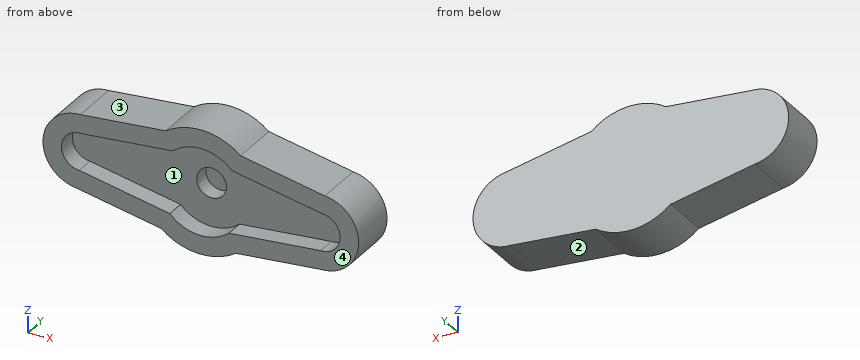
```python
from build123d import *

# Parameters (mm, degrees)
SKETCH1_R           = 2.032
BOSS_EXTRUDE1_DEPTH = 2.159
BOSS_EXTRUDE2_START = -2.54
BOSS_EXTRUDE2_DEPTH = 2.54
BOSS_EXTRUDE3_START = 2.159
BOSS_EXTRUDE3_DEPTH = 2


with BuildPart() as part:
    # Sketch1 → Boss-Extrude1 (new body)
    with BuildSketch(Plane(origin=(0, 19.05, 0), x_dir=(1, 0, 0), z_dir=(0, 1, 0))):
        with BuildLine():
            Line((27.891662372, 5.862371385), (16.22825993, 6.965475496))
            ThreePointArc((16.22825993, 6.965475496), (11.029140385, 8.448695687), (5.993806888, 6.479888246))
            Line((5.993806888, 6.479888246), (-5.512759891, 4.277454099))
            ThreePointArc((-5.512759891, 4.277454099), (-10.135739741, -1.023215233), (-5.031662372, -5.862371385))
            Line((-5.031662372, -5.862371385), (6.63174007, -6.965475496))
            ThreePointArc((6.63174007, -6.965475496), (11.830859615, -8.448695687), (16.866193112, -6.479888246))
            Line((16.866193112, -6.479888246), (28.372759891, -4.277454099))
            ThreePointArc((28.372759891, -4.277454099), (32.995739741, 1.023215233), (27.891662372, 5.862371385))
        make_face()
        with Locations(Location((11.43, 0, 0), (0, 0, 270))):
            Circle(SKETCH1_R, mode=Mode.SUBTRACT)
    extrude(amount=BOSS_EXTRUDE1_DEPTH)

    # Sketch1<3> → Boss-Extrude2 (add)
    with BuildSketch(Plane(origin=(0, 19.05, 0), x_dir=(1, 0, 0), z_dir=(0, 1, 0)).offset(BOSS_EXTRUDE2_START)):
        with BuildLine():
            Line((5.993806888, 6.479888246), (-5.512759891, 4.277454099))
            ThreePointArc((-5.512759891, 4.277454099), (-10.135739741, -1.023215233), (-5.031662372, -5.862371385))
            Line((-5.031662372, -5.862371385), (6.63174007, -6.965475496))
            ThreePointArc((6.63174007, -6.965475496), (11.830859615, -8.448695687), (16.866193112, -6.479888246))
            Line((16.866193112, -6.479888246), (28.372759891, -4.277454099))
            ThreePointArc((28.372759891, -4.277454099), (32.995739741, 1.023215233), (27.891662372, 5.862371385))
            Line((27.891662372, 5.862371385), (16.22825993, 6.965475496))
            ThreePointArc((16.22825993, 6.965475496), (11.029140385, 8.448695687), (5.993806888, 6.479888246))
        make_face()
        with BuildLine():
            ThreePointArc((28.0418263, -1.754687144), (30.458593889, 0.90283697), (27.801069775, 3.319604559))
            Line((27.801069775, 3.319604559), (15.268026397, 4.504957782))
            ThreePointArc((15.268026397, 4.504957782), (11.149518648, 5.911549835), (7.18268751, 4.121338114))
            Line((7.18268751, 4.121338114), (-5.1818263, 1.754687144))
            ThreePointArc((-5.1818263, 1.754687144), (-7.598593889, -0.90283697), (-4.941069775, -3.319604559))
            Line((-4.941069775, -3.319604559), (7.591973603, -4.504957782))
            ThreePointArc((7.591973603, -4.504957782), (11.710481352, -5.911549835), (15.67731249, -4.121338114))
            Line((15.67731249, -4.121338114), (28.0418263, -1.754687144))
        make_face(mode=Mode.SUBTRACT)
    extrude(amount=BOSS_EXTRUDE2_DEPTH)

    # Sketch1<4> → Boss-Extrude3 (add)
    with BuildSketch(Plane(origin=(0, 19.05, 0), x_dir=(1, 0, 0), z_dir=(0, 1, 0)).offset(BOSS_EXTRUDE3_START)):
        with BuildLine():
            Line((27.891662372, 5.862371385), (16.22825993, 6.965475496))
            ThreePointArc((16.22825993, 6.965475496), (11.029140385, 8.448695687), (5.993806888, 6.479888246))
            Line((5.993806888, 6.479888246), (-5.512759891, 4.277454099))
            ThreePointArc((-5.512759891, 4.277454099), (-10.135739741, -1.023215233), (-5.031662372, -5.862371385))
            Line((-5.031662372, -5.862371385), (6.63174007, -6.965475496))
            ThreePointArc((6.63174007, -6.965475496), (11.830859615, -8.448695687), (16.866193112, -6.479888246))
            Line((16.866193112, -6.479888246), (28.372759891, -4.277454099))
            ThreePointArc((28.372759891, -4.277454099), (32.995739741, 1.023215233), (27.891662372, 5.862371385))
        make_face()
    extrude(amount=BOSS_EXTRUDE3_DEPTH)


solid = part.part
```
Design review of the part built by this model. Coordinates are the model's own, in mm. Face numbers are marked on the shaded views. Give positions to 0.01 mm unless a question says otherwise; leave off trailing zeros. Order: outer loops, then holes, each group sorted by start corner. A loop starts at its lowest first (then second) coordinate and runs counter-clockwise, first axis right, second up. Notation, with made-up numbers: M -8.5,43 L 41.5,43 A9 ccw 41.5,59 Z; hole C 30.5,24 d3. An arc over 180 degrees is marked long. One line per question, with ' | ' between items. Start each with the question number.
Q1. We need section A-A (y = 19.5). Write out the cut boundary in (x, z).
Q2. For L1, parallel to Y at x = 27, z = 1.75; L2, parallel to Z at x = 5, y = 19; L3, parallel to Z at x = 3.5, y = 17, list the stretches that pass through material, from the lowest coordinate up. Write a range as [from, to].
Q3. For pin 1 Ø6 at (x, z) = (17, -2.5) entering from -Y; pin 2 Ø1.5 at (x, y) = (12.5, 21) entering from -Z; pin 3 Ø1.2 at (x, z) = (11, -0.5) entering from -Y, all flat-tipped, find the tip position at first contact; note any pin that passes through.
Q4. We need section B-B (y = 22.5). Write out the cut boundary in (x, z), plus the area to 3 significant figures.
Q5. We need section D-D (y = 17.75). Write out the cut boundary in (x, z).
Q6. We need section C-C (x = 11.43). Write out the cut boundary in (y, z), plus the area to 3 significant figures.
Q7. The part is to be moulded in two halves that separate along X. For the marked faces 1, 2, 3 and 4, say which applies: +X half, -X half, draft (parallel to the pull), parting line (faces both ways), or undercut.
Returned:
1) outline: M -5.51,-4.28 L 5.99,-6.48 A8.46 ccw 16.23,-6.97 L 27.89,-5.86 A5.08 ccw 28.37,4.28 L 16.87,6.48 A8.46 ccw 6.63,6.97 L -5.03,5.86 A5.08 ccw Z; hole C 11.43,0 d4.06
2) L1: [19.05, 23.21] | L2: [-6.29, -3.7], [4.26, 6.81] | L3: [-6, -3.42], [4.12, 6.67]
3) pin 1: y = 16.51 | pin 2: z = -8.45 | pin 3: y = 21.21
4) outline: M -5.51,-4.28 L 5.99,-6.48 A8.46 ccw 16.23,-6.97 L 27.89,-5.86 A5.08 ccw 28.37,4.28 L 16.87,6.48 A8.46 ccw 6.63,6.97 L -5.03,5.86 A5.08 ccw Z | area: 513 mm2
5) outline: M -5.51,-4.28 L 5.99,-6.48 A8.46 ccw 16.23,-6.97 L 27.89,-5.86 A5.08 ccw 28.37,4.28 L 16.87,6.48 A8.46 ccw 6.63,6.97 L -5.03,5.86 A5.08 ccw Z; hole M -5.18,-1.75 L 7.18,-4.12 A5.92 ccw 15.27,-4.5 L 27.8,-3.32 A2.54 ccw 28.04,1.75 L 15.68,4.12 A5.92 ccw 7.59,4.5 L -4.94,3.32 A2.54 ccw Z
6) outline: M 16.51,-8.46 L 23.21,-8.46 L 23.21,8.46 L 16.51,8.46 L 16.51,5.92 L 19.05,5.92 L 19.05,2.03 L 21.21,2.03 L 21.21,-2.03 L 19.05,-2.03 L 19.05,-5.92 L 16.51,-5.92 Z | area: 74.5 mm2
7) face 1: undercut | face 2: +X half | face 3: -X half | face 4: draft
